from build123d import *

# Parameters (mm, degrees)
CROQUIS1_W              = 9
CROQUIS1_H              = 20
CROQUIS1_R              = 1.7
SALIENTE_EXTRUIR1_DEPTH = 3
CORTAR_EXTRUIR2_DEPTH   = 1.5
CORTAR_EXTRUIR3_REACH   = 11
CROQUIS3_W              = 7
CROQUIS3_H              = 1
REDONDEO1_R             = 1
CROQUIS4_W              = 9
CROQUIS4_H              = 7
SALIENTE_EXTRUIR2_DEPTH = 0.3


with BuildPart() as part:
    # Croquis1 → Saliente-Extruir1 (new body)
    with BuildSketch(Plane(origin=(0, 0, 0), x_dir=(1, 0, 0), z_dir=(0, 1, 0))):
        with Locations((165.454426616, -12)):
            Rectangle(CROQUIS1_W, CROQUIS1_H)
        with Locations((165.962302832, -4.25)):
            Circle(CROQUIS1_R, mode=Mode.SUBTRACT)
        with Locations((165.962302832, -19.75)):
            Circle(CROQUIS1_R, mode=Mode.SUBTRACT)
    extrude(amount=-SALIENTE_EXTRUIR1_DEPTH)

    # Croquis2 → Cortar-Extruir2 (cut)
    with BuildSketch(Plane.XZ.offset(3)):
        Polygon((168.943819954, 21.471379713), (165.962302832, 23.192759426), (162.98078571, 21.471379713), (162.98078571, 18.028620287), (165.962302832, 16.307240574), (168.943819954, 18.028620287), align=None)
        Polygon((168.943819954, 5.971379713), (168.943819954, 2.528620287), (165.962302832, 0.807240574), (162.98078571, 2.528620287), (162.98078571, 5.971379713), (165.962302832, 7.692759426), align=None)
    extrude(amount=-CORTAR_EXTRUIR2_DEPTH, mode=Mode.SUBTRACT)

    # Croquis3 → Cortar-Extruir3 (cut, up to next)
    with BuildSketch(Plane.ZY.offset(-160.954426616), mode=Mode.PRIVATE) as cortar_extruir3_sk1:
        with Locations((12, -0.5)):
            Rectangle(CROQUIS3_W, CROQUIS3_H)
    cortar_extruir3_tool1 = extrude(cortar_extruir3_sk1.sketch, amount=-CORTAR_EXTRUIR3_REACH, mode=Mode.PRIVATE) & part.part
    add(cortar_extruir3_tool1.solids().sort_by_distance((160.954427, -0.5, 12))[0], mode=Mode.SUBTRACT)

    # Redondeo1
    redondeo1_edges = [part.edges().sort_by_distance(p)[0] for p in [
        (160.954426616, -3, 12),
        (160.954426616, -1.5, 2),
        (160.954426616, -1.5, 22),
    ]]
    fillet(redondeo1_edges, radius=REDONDEO1_R)

    # Croquis4 → Saliente-Extruir2 (add)
    with BuildSketch(Plane(origin=(0, -1, 0), x_dir=(1, 0, 0), z_dir=(0, 1, 0))):
        with Locations((165.454426616, -12)):
            Rectangle(CROQUIS4_W, CROQUIS4_H)
    extrude(amount=SALIENTE_EXTRUIR2_DEPTH)


solid = part.part
Work out the finished part from the listing and answer in its coordinate system (mm). A direction names the side the tool comes from. Give positions to 0.01 mm unless a question says otherwise; leave off trailing zeros. Write each loop counter-clockwise with the first axis right and the second up, starting at its lowest first coordinate (ties: lowest second). Pieces come first, ordered by that corner, then holes. Notation, with made-up numbers: (70, 89.5) - (115, 89.5) arc R35 ccw to (115, 122.5) - close; hole circle Ø1 at (-1, 54.25). An arc over 180 degrees is marked (long way). One line per item, written item: value. Start each with the question number.
1. Consider probe 1 along X at (y, z) = (-1, 4.25); probe 2 along Z at (x, y) = (165.5, -1.15); probe 3 along Z at (x, y) = (165, -0.65). Determine where each line is inside the solid, lowest interval first.
2. Find section D-D (z = 9). Write down the section's boundary in (x, y), then the cut area to 3 significant figures.
3. Find section B-B (y = -0.35). Write down the section's boundary in (x, z).
4. Find section C-C (x = 167.25). Write down the section's boundary in (y, z), then the cut area to 3 significant figures.
5. Given pin 1 (2 mm diameter, centred on x = 165, z = 12, fed in from +Y); pin 2 (2 mm diameter, centred on x = 166, z = 7.5, fed in from +Y); pin 3 (3 mm diameter, centred on x = 166, z = 5, fed in from -Y); pin 4 (2.5 mm diameter, centred on x = 165.96, z = 4.25, fed in from +Y), each flat-ended and moving along its own axis, determine where each tip first touches the part or whether it passes through.
6. For faces 1 (the flat face through (165, 0, 18)), 2 (the flat face through (165, -1.5, 6)), determine the directions among +Z, -Z, +X, -X, +Y, -Y from which every point of the face is accessible in a straight line to the end or side of a thin tool.
7. For a pull along X with two mould halves and no side action, classify faces 3 (the cylindrical face through (161.24, -1.52, 2.3)), 4 (the flat face through (166, -3, 12)), 5 (the flat face through (163.445, -2.26, 2.261)) as +X half, -X half, draft (parallel to the pull), parting line (faces both ways), or undercut.
8. Find section A-A (z = 19.75). Write down the section's boundary in (x, y).
Geometry results:
1. probe 1: 160.95 to 164.26, 167.66 to 169.95
1. probe 2: 2 to 2.61, 5.89 to 18.11, 21.39 to 22
1. probe 3: 2 to 2.85, 5.65 to 8.5, 15.5 to 18.35, 21.15 to 22
2. outline: (160.95, -2) arc R1 ccw to (161.95, -3) - (169.95, -3) - (169.95, -0.7) - (160.95, -0.7) - close
2. area: 20.5 mm2
3. outline: (160.95, 3) arc R1 ccw to (161.95, 2) - (169.95, 2) - (169.95, 8.5) - (160.95, 8.5) - close; (160.95, 15.5) - (169.95, 15.5) - (169.95, 22) - (161.95, 22) arc R1 ccw to (160.95, 21) - close; hole circle Ø3.4 at (165.96, 4.25); hole circle Ø3.4 at (165.96, 19.75)
4. outline: (-3, 6.95) - (-1.5, 6.95) - (-1.5, 5.36) - (0, 5.36) - (0, 8.5) - (-0.7, 8.5) - (-0.7, 15.5) - (0, 15.5) - (0, 18.64) - (-1.5, 18.64) - (-1.5, 17.05) - (-3, 17.05) - close; (-1.5, 2) - (0, 2) - (0, 3.14) - (-1.5, 3.14) - close; (-1.5, 20.86) - (0, 20.86) - (0, 22) - (-1.5, 22) - close
4. area: 33.6 mm2
5. pin 1: y = -0.7
5. pin 2: y = 0
5. pin 3: y = -1.5
5. pin 4: through
6. face 1: +Z, -Z, +X, -X, +Y
6. face 2: -Y
7. face 3: -X half
7. face 4: draft
7. face 5: undercut
8. outline: (160.95, -2) arc R1 ccw to (161.95, -3) - (162.98, -3) - (162.98, -1.5) - (164.26, -1.5) - (164.26, 0) - (160.95, 0) - close; (167.66, -1.5) - (168.94, -1.5) - (168.94, -3) - (169.95, -3) - (169.95, 0) - (167.66, 0) - close
